Drawing for the job (mm, zero at the part's lowest x, y, z). Give positions to 0.01 mm unless a question says otherwise; leave off trailing zeros. Loops run counter-clockwise (first coordinate to the right, second up) from the corner with the lowest first, then second, coordinate; pieces in that order, holes last. Notation, with made-up numbers: (40.5, -2.5) -> (94.5, -2.5) arc R9 cw to (94.5, 2.5) -> close; hole circle Ø7 at (40, 83.25). An arc over 180 degrees is marked (long way). Use CSV: the item, a comma, the result in double quotes. Start each with the question number.
(1) Cut at B-B on y = 36. Write the cut outline in (x, z), then the cut area to 3 significant figures.
(2) Cut at A-A on x = 46. Write the cut outline in (y, z).
(3) Cut at D-D on x = 32.6. Write the cut outline in (y, z).
(4) Cut at C-C on z = 2.1. State how many separate pieces and enclosed holes the cut face has, then the cut area to 3 significant figures.
(5) Drill centre lines: probe 1 along Y at (x, z) = (32.6, 2.05); probe 2 along Y at (x, z) = (45.5, 0.85); probe 3 along X at (y, z) = (41.5, 2.4). Where is each one in solid material? Low to high.
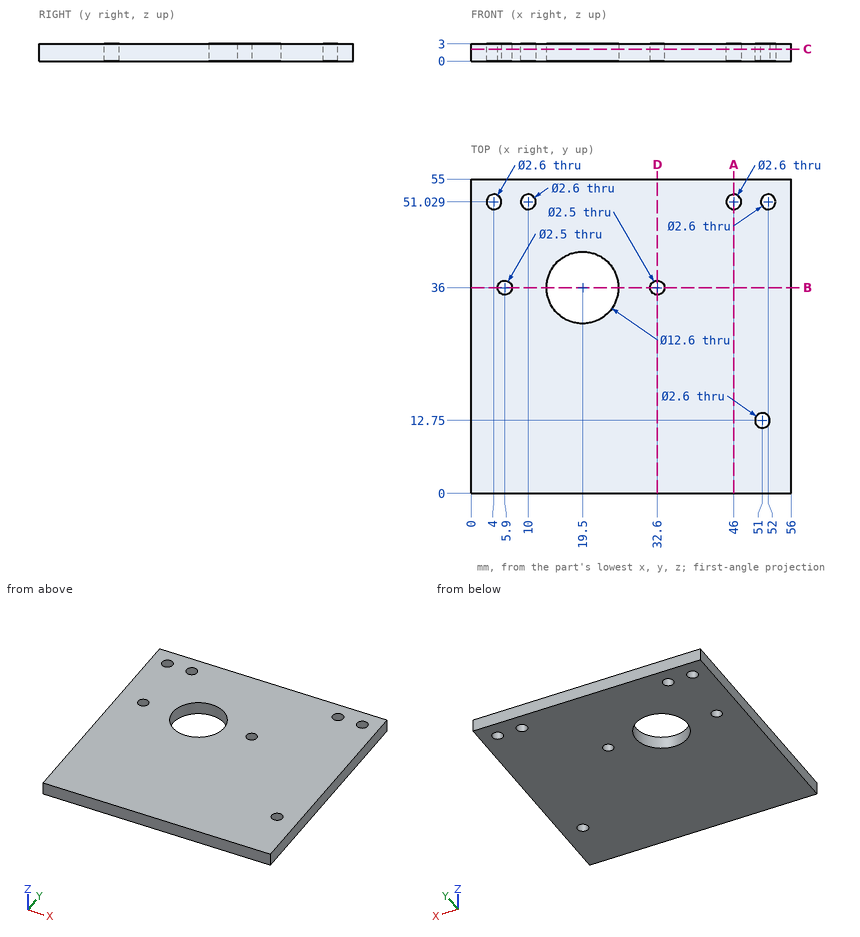
Check result:
1,outline,"(0, 0) -> (4.65, 0) -> (4.65, 3) -> (0, 3) -> close; (7.15, 0) -> (13.2, 0) -> (13.2, 3) -> (7.15, 3) -> close; (25.8, 0) -> (31.35, 0) -> (31.35, 3) -> (25.8, 3) -> close; (33.85, 0) -> (56, 0) -> (56, 3) -> (33.85, 3) -> close"
1,area,"115 mm²"
2,outline,"(0, 0) -> (49.73, 0) -> (49.73, 3) -> (0, 3) -> close; (52.33, 0) -> (55, 0) -> (55, 3) -> (52.33, 3) -> close"
3,outline,"(0, 0) -> (34.75, 0) -> (34.75, 3) -> (0, 3) -> close; (37.25, 0) -> (55, 0) -> (55, 3) -> (37.25, 3) -> close"
4,separate pieces,"1"
4,enclosed holes,"8"
4,area,"2,920 mm²"
5,probe 1,"0 to 34.75, 37.25 to 55"
5,probe 2,"0 to 49.83, 52.23 to 55"
5,probe 3,"0 to 16.43, 22.57 to 56"
